For this review, take the finished solid that the model builds, in its own axes (mm). Face numbers are marked on the shaded views. A direction names the side the tool comes from. Round coordinates to 2 decimals unless told otherwise and drop trailing zeros. Write each loop counter-clockwise with the first axis right and the second up, starting at its lowest first coordinate (ties: lowest second). Pieces come first, ordered by that corner, then holes. Notation, with made-up numbers: (89.25, -33) -> (114.25, -33) arc R13 ccw to (114.25, -20) -> close; hole circle Ø5 at (54.25, 47.5). An arc over 180 degrees is marked (long way). Answer in a Markdown table with one row per item.
from build123d import *

# Parameters (mm, degrees)
SKETCH_R        = 10
SKETCH_R_2      = 4.7
PAD_DEPTH       = 30
SKETCH001_R     = 5.85
POCKET_DEPTH    = 10
POCKET001_DEPTH = 11
SKETCH003_R     = 2.25
POCKET002_DEPTH = 13
FILLET_R        = 1


with BuildPart() as part:
    # Sketch → Pad (new body)
    with BuildSketch(Plane.XY):
        Circle(SKETCH_R)
        Circle(SKETCH_R_2, mode=Mode.SUBTRACT)
    extrude(amount=PAD_DEPTH)

    # Sketch001 → Pocket (cut)
    with BuildSketch(Plane.XY):
        Circle(SKETCH001_R)
    extrude(amount=POCKET_DEPTH, mode=Mode.SUBTRACT)

    # Sketch002 → Pocket001 (cut, symmetric)
    with BuildSketch(Plane.XZ):
        with BuildLine():
            ThreePointArc((5.85, 10), (0, 15.85), (-5.85, 10))
            Line((-5.85, 10), (-5.85, 0))
            Line((-5.85, 0), (5.85, 0))
            Line((5.85, 0), (5.85, 10))
        make_face()
    extrude(amount=POCKET001_DEPTH, both=True, mode=Mode.SUBTRACT)

    # Sketch003 (on DatumPlane) → Pocket002 (cut, symmetric)
    with BuildSketch(Plane(origin=(0, 0, 0), x_dir=(0, -1, 0), z_dir=(-1, 0, 0))):
        with Locations((0, 5)):
            Circle(SKETCH003_R)
    extrude(amount=POCKET002_DEPTH, both=True, mode=Mode.SUBTRACT)

    # Fillet
    fillet_edges = [part.edges().sort_by_distance(p)[0] for p in [
        (-10, 0, 0),
        (8.902247, 4.555217, 0),
        (8.902247, -4.555217, 0),
    ]]
    fillet(fillet_edges, radius=FILLET_R)


solid = part.part
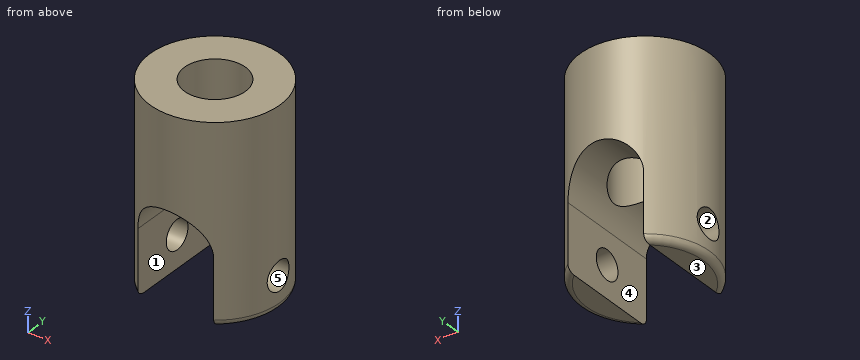
1) Consider section D-D on z = 14. State the section outline as (x, y) points, then the cut area to 3 significant figures.
Solved:
| item | result |
|---|---|
| outline | (-4.27, -9.04) -> (-4.27, -1.97) arc R4.7 cw to (-4.27, 1.97) -> (-4.27, 9.04) arc R10 ccw to start; (4.27, -9.04) arc R10 ccw to (4.27, 9.04) -> (4.27, 1.97) arc R4.7 cw to (4.27, -1.97) -> close |
| area | 146 mm² |
2) Consider section B-B on x = 0. State the section outline as (y, z) points, then the cut area to 3 significant figures.
Solved:
| item | result |
|---|---|
| outline | (-10, 15.85) -> (-4.7, 15.85) -> (-4.7, 30) -> (-10, 30) -> close; (4.7, 15.85) -> (10, 15.85) -> (10, 30) -> (4.7, 30) -> close |
| area | 150 mm² |
3) Clearance check with flat-ended pins moving along their axes: pin 1 Ø4 at (y, z) = (-3.5, 21) entering from +X; pin 2 Ø1 at (x, z) = (-3, 25.5) entering from +Y; pin 3 Ø4 at (x, y) = (1.5, 6.5) entering from -Z. State where each tip first meets the part, or that it passes through.
Solved:
| item | result |
|---|---|
| pin 1 | x = 9.89 |
| pin 2 | y = 9.68 |
| pin 3 | z = 14.69 |
4) Consider section A-A on y = 0. State the section outline as (x, z) points, then the cut area to 3 significant figures.
Solved:
| item | result |
|---|---|
| outline | (-10, 1) arc R1 ccw to (-9, 0) -> (-5.85, 0) -> (-5.85, 2.75) -> (-10, 2.75) -> close; (-10, 7.25) -> (-5.85, 7.25) -> (-5.85, 10) arc R5.85 cw to (-4.7, 13.48) -> (-4.7, 30) -> (-10, 30) -> close; (4.7, 13.48) arc R5.85 cw to (5.85, 10) -> (5.85, 7.25) -> (10, 7.25) -> (10, 30) -> (4.7, 30) -> close; (5.85, 0) -> (9, 0) arc R1 ccw to (10, 1) -> (10, 2.75) -> (5.85, 2.75) -> close |
| area | 252 mm² |
5) Mouldability with a two-part tool opening along Z and no side actions: class the marked faces 1, 2 and 3 as pulls with the +Z half, pulls with the -Z half, needs draft (parallel to the pull), parting line crosses it, or undercut.
Solved:
| item | result |
|---|---|
| face 1 | needs draft |
| face 2 | undercut |
| face 3 | pulls with the -Z half |
6) For the marked faces 4 and 5, list the 3-axis set-ups (+Z, -Z, +X, -X, +Y, -Y) from which the entire face can be reached by the end or side of a thin tool; tool diameter is ignored.
Solved:
| item | result |
|---|---|
| face 4 | -Z, +Y, -Y |
| face 5 | +X, -X |
7) Consider section C-C on z = 5. State the section outline as (x, y) points, then the cut area to 3 significant figures.
Solved:
| item | result |
|---|---|
| outline | (-9.74, -2.25) arc R10 ccw to (-5.85, -8.11) -> (-5.85, -2.25) -> close; (-9.74, 2.25) -> (-5.85, 2.25) -> (-5.85, 8.11) arc R10 ccw to start; (5.85, -8.11) arc R10 ccw to (9.74, -2.25) -> (5.85, -2.25) -> close; (5.85, 2.25) -> (9.74, 2.25) arc R10 ccw to (5.85, 8.11) -> close |
| area | 57.7 mm² |
8) For line 1 (X direction, y = 0, z = 17); line 2 (Z direction, x = 7.35, y = 0), list the stretches that pass through material, from the lowest coordinate up. Write a range as [from, to].
Solved:
| item | result |
|---|---|
| line 1 | [-10, -4.7], [4.7, 10] |
| line 2 | [0, 2.75], [7.25, 30] |
